Could you check a few things on this model? Use its own coordinates, in mm. Face numbers are marked on the shaded views. A direction names the side the tool comes from. Give positions to 0.01 mm unless a question says otherwise; leave off trailing zeros. Loops run counter-clockwise (first coordinate to the right, second up) from the corner with the lowest first, then second, coordinate; pieces in that order, holes last. Notation, with made-up numbers: (6, -36) -> (35, -36) arc R23 cw to (35, -9) -> close; hole circle Ø2 at (-6.75, 78). An arc over 180 degrees is marked (long way). Write item = value, one per line. Start each with the question number.
1) I want a section at A-A (y = 9.25). List the corners of the cut face in (x, z) for me, and give its area (3 significant figures).
2) I want a section at D-D (z = -43.5). List the corners of the cut face in (x, y) for me (3 decimals).
3) I want a section at C-C (z = 67). List the corners of the cut face in (x, y) for me.
4) On a 3-axis mill with a long thin cutter (end or side, diameter ignored), from which of +Z, -Z, +X, -X, +Y, -Y can I reach the whole of each face in a straight line? I mean the marked faces 1 and 2. Say none if no direction works.
5) I'm going to push flat-ended pins straight in: pin 1 Ø2 at (x, y) = (7.5, 9.5) entering from +Z; pin 2 Ø3.5 at (x, z) = (-7, 73) entering from -Y; pin 3 Ø4 at (x, y) = (-15, 8.5) entering from -Z. Where does each tip first touch, or does it pass through?
6) I need wall thicknesses on probe 1 along X at (y, z) = (8, 74.5); probe 2 along X at (y, z) = (3.75, -85); probe 3 along Z at (x, y) = (-5, 8.5). Which ranges of each line are inside material? Lowest first, please. Write a range as from..to.
7) I want a section at B-B (z = 45). List the corners of the cut face in (x, y) for me.
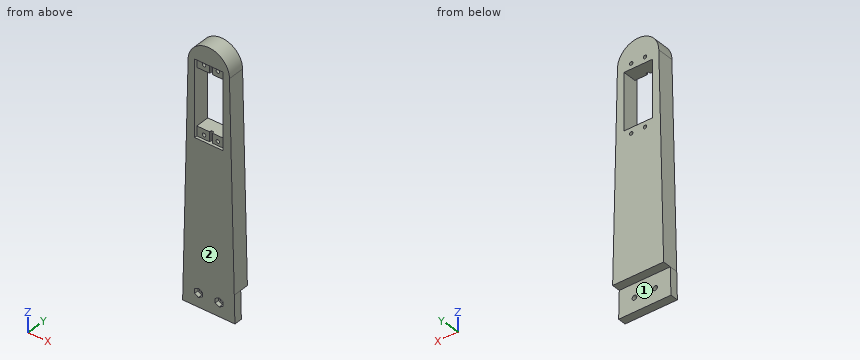
from build123d import *

# Parameters (mm, degrees)
BOSS_EXTRUDE1_DEPTH = 12
BOSS_EXTRUDE2_DEPTH = 5.9
SKETCH3_R           = 1.7
CUT_EXTRUDE1_DEPTH  = 5.9
CUT_EXTRUDE2_DEPTH  = 3
SKETCH5_W           = 20.5
SKETCH5_H           = 41
CUT_EXTRUDE3_DEPTH  = 12
SKETCH6_W           = 20.5
SKETCH6_H           = 55
CUT_EXTRUDE4_DEPTH  = 2
SKETCH7_W           = 2
SKETCH7_H           = 7
CUT_EXTRUDE5_DEPTH  = 1.5
SKETCH8_R           = 1.25
CUT_EXTRUDE6_DEPTH  = 12


with BuildPart() as part:
    # Sketch1 → Boss-Extrude1 (new body)
    with BuildSketch(Plane(origin=(0, 0, 0), x_dir=(1, 0, 0), z_dir=(0, 1, 0))):
        with BuildLine():
            Line((18.5, 75), (-18.5, 75))
            Line((-18.5, 75), (-15, -75))
            ThreePointArc((-15, -75), (0, -90), (15, -75))
            Line((15, -75), (18.5, 75))
        make_face()
    extrude(amount=BOSS_EXTRUDE1_DEPTH)

    # Sketch2 → Boss-Extrude2 (add)
    with BuildSketch(Plane.XZ):
        Polygon((-18.965, -95), (18.965, -95), (18.5, -75), (-18.5, -75), align=None)
        with BuildLine():
            Line((-18.5, -75), (18.5, -75))
            Line((18.5, -75), (15, 75))
            ThreePointArc((15, 75), (0, 90), (-15, 75))
            Line((-15, 75), (-18.5, -75))
        make_face()
    extrude(amount=-BOSS_EXTRUDE2_DEPTH)

    # Sketch3 → Cut-Extrude1 (cut)
    with BuildSketch(Plane.XZ):
        with Locations((-7.5, -85)):
            Circle(SKETCH3_R)
        with Locations((7.5, -85)):
            Circle(SKETCH3_R)
    extrude(amount=-CUT_EXTRUDE1_DEPTH, mode=Mode.SUBTRACT)

    # Sketch4 → Cut-Extrude2 (cut)
    with BuildSketch(Plane.XZ):
        Polygon((-7.5, -81.766838493), (-10.3, -83.383419246), (-10.3, -86.616580754), (-7.5, -88.233161507), (-4.7, -86.616580754), (-4.7, -83.383419246), align=None)
        Polygon((7.5, -81.766838493), (4.7, -83.383419246), (4.7, -86.616580754), (7.5, -88.233161507), (10.3, -86.616580754), (10.3, -83.383419246), align=None)
    extrude(amount=-CUT_EXTRUDE2_DEPTH, mode=Mode.SUBTRACT)

    # Sketch5 → Cut-Extrude3 (cut)
    with BuildSketch(Plane.XZ):
        with Locations((0, 50)):
            Rectangle(SKETCH5_W, SKETCH5_H)
    extrude(amount=-CUT_EXTRUDE3_DEPTH, mode=Mode.SUBTRACT)

    # Sketch6 → Cut-Extrude4 (cut)
    with BuildSketch(Plane.XZ):
        with Locations((0, 50)):
            Rectangle(SKETCH6_W, SKETCH6_H)
    extrude(amount=-CUT_EXTRUDE4_DEPTH, mode=Mode.SUBTRACT)

    # Sketch7 → Cut-Extrude5 (cut)
    with BuildSketch(Plane.XZ.offset(-2)):
        with Locations((0, 74)):
            Rectangle(SKETCH7_W, SKETCH7_H)
        with Locations((0, 26)):
            Rectangle(SKETCH7_W, SKETCH7_H)
    extrude(amount=-CUT_EXTRUDE5_DEPTH, mode=Mode.SUBTRACT)

    # Sketch8 → Cut-Extrude6 (cut)
    with BuildSketch(Plane.XZ.offset(-2)):
        with Locations((-5, 74.5)):
            Circle(SKETCH8_R)
        with Locations((5, 74.5)):
            Circle(SKETCH8_R)
        with Locations((5, 25.5)):
            Circle(SKETCH8_R)
        with Locations((-5, 25.5)):
            Circle(SKETCH8_R)
    extrude(amount=-CUT_EXTRUDE6_DEPTH, mode=Mode.SUBTRACT)


solid = part.part
Answer list:
q1.outline = (-18.5, -75) -> (18.5, -75) -> (15, 75) arc R15 ccw to (-15, 75) -> close; hole (-10.25, 29.5) -> (10.25, 29.5) -> (10.25, 70.5) -> (-10.25, 70.5) -> close; hole circle Ø2.5 at (-5, 25.5); hole circle Ø2.5 at (-5, 74.5); hole circle Ø2.5 at (5, 25.5); hole circle Ø2.5 at (5, 74.5)
q1.area = 4,520 mm^2
q2.outline = (-17.765, 0) -> (17.765, 0) -> (17.765, 12) -> (-17.765, 12) -> close
q3.outline = (-15.19, 0) -> (-10.25, 0) -> (-10.25, 12) -> (-15.19, 12) -> close; (10.25, 0) -> (15.19, 0) -> (15.19, 12) -> (10.25, 12) -> close
q4.face_1 = -Z, +X, -X, +Y
q4.face_2 = +Z, -Z, +X, -X, -Y
q5.pin_1 = 88.52
q5.pin_2 = 2
q5.pin_3 = -75
q6.probe_1 = -15.01..-6.25, -3.75..3.75, 6.25..15.01
q6.probe_2 = -18.73..-9.2, -5.8..5.8, 9.2..18.73
q6.probe_3 = -75..24.25, 26.75..29.5, 70.5..73.25, 75.75..89.14
q7.outline = (-15.7, 0) -> (-10.25, 0) -> (-10.25, 12) -> (-15.7, 12) -> close; (10.25, 0) -> (15.7, 0) -> (15.7, 12) -> (10.25, 12) -> close
